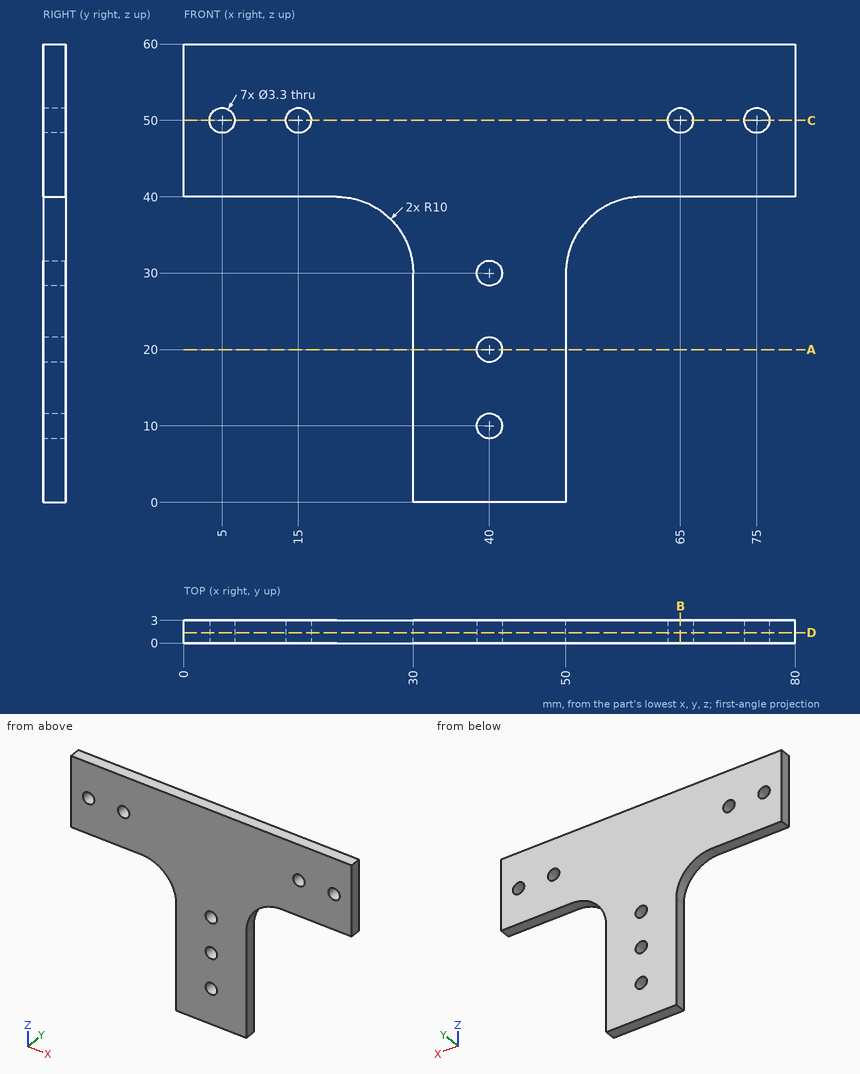
Verification items for this drawing (mm, ordinates from the low corner). Round coordinates to 2 decimals unless told otherwise and drop trailing zeros. Loops run counter-clockwise (first coordinate to the right, second up) from the corner with the lowest first, then second, coordinate; pieces in that order, holes last. Notation, with made-up numbers: M 80,55.5 L 102,55.5 A22 ccw 102,77.5 Z; hole C 17,88 d1. An arc over 180 degrees is marked long. Answer as a JSON object with one key per item and string values.
1. Gauge pin test, flat ends, axial feed: P1, Ø1.5, axis at y = 2, z = 16.5, coming from the +X side; P2, Ø2, axis at x = 40, z = 10, coming from the +Y side; P3, Ø1.5, axis at x = 74, y = 2, coming from the -Z side. Record the tip position at first contact, or that the pin passes through.
Reply:
{"P1": "stops at x = 50", "P2": "passes through", "P3": "stops at z = 40"}
2. Section check C-C (z = 50). Record the boundary of the cut face in (x, y), plus the area to 3 significant figures.
Reply:
{"outline": "M 0,0 L 3.35,0 L 3.35,3 L 0,3 Z; M 6.65,0 L 13.35,0 L 13.35,3 L 6.65,3 Z; M 16.65,0 L 63.35,0 L 63.35,3 L 16.65,3 Z; M 66.65,0 L 73.35,0 L 73.35,3 L 66.65,3 Z; M 76.65,0 L 80,0 L 80,3 L 76.65,3 Z", "area": "200 mm²"}
3. Section check D-D (y = 1.4). Record the boundary of the cut face in (x, z).
Reply:
{"outline": "M 0,40 L 20,40 A10 cw 30,30 L 30,0 L 50,0 L 50,30 A10 cw 60,40 L 80,40 L 80,60 L 0,60 Z; hole C 5,50 d3.3; hole C 15,50 d3.3; hole C 40,10 d3.3; hole C 40,20 d3.3; hole C 40,30 d3.3; hole C 65,50 d3.3; hole C 75,50 d3.3"}
4. Section check B-B (x = 65). Record the boundary of the cut face in (y, z).
Reply:
{"outline": "M 0,40 L 3,40 L 3,48.35 L 0,48.35 Z; M 0,51.65 L 3,51.65 L 3,60 L 0,60 Z"}
5. Scan lines: line 1 (X direction, y = 1.4, z = 50); line 2 (Z direction, x = 75, y = 1.95); line 3 (X direction, y = 2.25, z = 10). Record each from-to range of solid material in increasing order.
Reply:
{"line 1": "x = 0 to 3.35, 6.65 to 13.35, 16.65 to 63.35, 66.65 to 73.35, 76.65 to 80", "line 2": "z = 40 to 48.35, 51.65 to 60", "line 3": "x = 30 to 38.35, 41.65 to 50"}
6. Section check A-A (z = 20). Record the boundary of the cut face in (x, y), plus the area to 3 significant figures.
Reply:
{"outline": "M 30,0 L 38.35,0 L 38.35,3 L 30,3 Z; M 41.65,0 L 50,0 L 50,3 L 41.65,3 Z", "area": "50.1 mm²"}
